Input: part model. Units: mm. Frame: model coordinates. A direction names the side the tool comes from. Give positions to 0.01 mm unless a question says otherwise; leave off trailing zeros. Order: outer loops, then holes, each group sorted by start corner. A loop starts at its lowest first (then second) coordinate and runs counter-clockwise, first axis right, second up. Notation, with made-up numbers: (28.5, 2) - (64.5, 2) arc R22 cw to (64.5, 31) - close; hole circle Ø7 at (55.25, 18). An arc over 180 degrees is marked (long way). Use a Markdown table: item, result.
from build123d import *

# Parameters (mm, degrees)
F0_W     = 406.4
F0_H     = 203.2
F0_W_2   = 146.05
F0_H_2   = 127
F1_DEPTH = 203.2


with BuildPart() as f1:
    # F0 (on Front) → F1 (new body)
    with BuildSketch(Plane.XZ):
        Rectangle(F0_W, F0_H)
        with Locations((-92.075, 0)):
            Rectangle(F0_W_2, F0_H_2, mode=Mode.SUBTRACT)
        with Locations((92.075, 0)):
            Rectangle(F0_W_2, F0_H_2, mode=Mode.SUBTRACT)
    extrude(amount=-F1_DEPTH)


solid = f1.part
1. Section query C-C (z = -37.5). Return loops of the section in (x, y), then the cut area to 3 significant figures.
Response:
| item | result |
|---|---|
| outline | (-203.2, 0) - (-165.1, 0) - (-165.1, 203.2) - (-203.2, 203.2) - close; (-19.05, 0) - (19.05, 0) - (19.05, 203.2) - (-19.05, 203.2) - close; (165.1, 0) - (203.2, 0) - (203.2, 203.2) - (165.1, 203.2) - close |
| area | 23,200 mm^2 |
2. Set-up query: faces 5 (the face through (91, 100, -63.5)), 6 (the face through (-3, 100, 101.6)). Return all of +Z, -Z, +X, -X, +Y, -Y with unobstructed straight access to the full face (end or side cutting, diameter ignored); none if empty.
Response:
| item | result |
|---|---|
| face 5 | +Y, -Y |
| face 6 | +Z, +X, -X, +Y, -Y |
3. Section query B-B (y = 136). Return loops of the section in (x, z).
Response:
| item | result |
|---|---|
| outline | (-203.2, -101.6) - (203.2, -101.6) - (203.2, 101.6) - (-203.2, 101.6) - close; hole (-165.1, -63.5) - (-19.05, -63.5) - (-19.05, 63.5) - (-165.1, 63.5) - close; hole (19.05, -63.5) - (165.1, -63.5) - (165.1, 63.5) - (19.05, 63.5) - close |
4. Material intervals for line 1 along X through (y, z) = (95, -45); line 2 along Z through (x, y) = (-80, 156.5), sorted ascending.
Response:
| item | result |
|---|---|
| line 1 | x = -203.2 to -165.1, -19.05 to 19.05, 165.1 to 203.2 |
| line 2 | z = -101.6 to -63.5, 63.5 to 101.6 |
5. Section query A-A (x = 76). Return loops of the section in (y, z).
Response:
| item | result |
|---|---|
| outline | (0, -101.6) - (203.2, -101.6) - (203.2, -63.5) - (0, -63.5) - close; (0, 63.5) - (203.2, 63.5) - (203.2, 101.6) - (0, 101.6) - close |
6. Mould query, pull axis Z, two halves, no side actions, for faces 1 (the face through (-93, 100, 63.5)), 2 (the face through (-3, 0, 1)), 3 (the face through (91, 100, 63.5)), 4 (the face through (-3, 100, -101.6)). Classes: pulls with the +Z half, pulls with the -Z half, needs draft (parallel to the pull), parting line crosses it, or undercut.
Response:
| item | result |
|---|---|
| face 1 | undercut |
| face 2 | needs draft |
| face 3 | undercut |
| face 4 | pulls with the -Z half |
